Check sheet for the modelled part. Datum: model origin and axes. Units: mm. A direction names the side the tool comes from. Round coordinates to 2 decimals unless told otherwise and drop trailing zeros. Write each loop counter-clockwise with the first axis right and the second up, starting at its lowest first coordinate (ties: lowest second). Pieces come first, ordered by that corner, then holes. Notation, with made-up numbers: (76.5, -15) - (96.5, -15) arc R32 cw to (96.5, 15) - close; hole circle Ø5 at (39, 8.25). An arc over 180 degrees is marked (long way). Use one line per item in the form item = value. Start each with the question number.
1) Section check B-B (x = -83). Record the boundary of the cut face in (y, z).
2) Draft check along X on faces 1 (the face through (-90.14, -37.35, 19.32)), 2 (the face through (-110, -44.45, 16)), 3 (the face through (-31.433, -22, 6)). Enter one of: +X half, -X half, draft (parallel to the pull), parting line (faces both ways), or undercut.
3) Gauge pin test, flat ends, axial feed: P1, Ø8, axis at x = -94, y = -3, coming from the +Z side; P2, Ø5, axis at x = -149, y = -14, coming from the +Z side; P3, Ø1.5, axis at x = -154.5, y = -14, coming from the -Z side. Record the tip position at first contact, or that the pin passes through.
4) Section check A-A (y = -17.5). Record the boundary of the cut face in (x, z) (1 decimal), then the cut area to 3 significant figures.
5) Section check C-C (x = -56.5). Record the boundary of the cut face in (y, z), then the cut area to 3 significant figures.
6) Set-up check for faces 4 (the face through (-134.144, -22, 2)), 5 (the face through (-166.804, -29.652, 29.227)), 6 (the face through (-104, -41, 7.62)), 7 (the face through (-80, -7.62, 7)), 8 (the face through (-126.524, -23, 12)): record each of +Z, -Z, +X, -X, +Y, -Y from which the full face is reachable in a straight line by a thin tool's end or side.
7) Scan lines: probe 1 along Y at (x, z) = (-123, 2); probe 2 along X at (y, z) = (-12, 15). Record each from-to range of solid material in increasing order.
8) Section check D-D (z = 22). Record the boundary of the cut face in (x, y), then the cut area to 3 significant figures.
from build123d import *

# Parameters (mm, degrees)
F0_W      = 177.8
F0_H      = 44.45
F1_DEPTH  = 31.75
F2_W      = 1.5875
F2_H      = 44.45
F3_DEPTH  = 3.175
F4_W      = 95.09125
F4_H      = 29.21
F5_DEPTH  = 31.751
F7_DEPTH  = 44.451
F9_DEPTH  = 44.451
F11_DEPTH = 44.451
F13_DEPTH = 177.801
F14_R     = 2.54


with BuildPart() as f1:
    # F0 (on Top) → F1 (new body)
    with BuildSketch(Plane.XY):
        with Locations((-88.9, -22.225)):
            Rectangle(F0_W, F0_H)
    extrude(amount=F1_DEPTH)

    # F2 (on face) → F3 (cut)
    with BuildSketch(Plane(origin=(0, 0, 0), x_dir=(1, 0, 0), z_dir=(0, 0, -1))):
        with Locations((-23.01875, 22.225)):
            Rectangle(F2_W, F2_H)
        with Locations((-134.9375, 22.225)):
            Rectangle(F2_W, F2_H)
    extrude(amount=-F3_DEPTH, mode=Mode.SUBTRACT)

    # F4 (on face) → F5 (cut, through all)
    with BuildSketch(Plane.XY.offset(31.75)):
        with Locations((-78.978125, -22.225)):
            Rectangle(F4_W, F4_H)
    extrude(amount=-F5_DEPTH, mode=Mode.SUBTRACT)

    # F6 (on face) → F7 (cut, through all)
    with BuildSketch(Plane.XZ.offset(44.45)):
        Polygon((-177.8, 31.75), (0, 6.540501), (0, 31.75), align=None)
    extrude(amount=-F7_DEPTH, mode=Mode.SUBTRACT)

    # F8 (on face) → F9 (cut, through all)
    with BuildSketch(Plane.XZ.offset(44.45)):
        with BuildLine():
            Line((-126.52375, 16.783548), (-126.52375, 7.62))
            Line((-126.52375, 7.62), (-79.898132, 7.62))
            ThreePointArc((-79.898132, 7.62), (-78.63128, 8.800636), (-79.719847, 10.147424))
            Line((-79.719847, 10.147424), (-126.52375, 16.783548))
        make_face()
    extrude(amount=-F9_DEPTH, mode=Mode.SUBTRACT)

    # F10 (on face) → F11 (cut, through all)
    with BuildSketch(Plane.XZ.offset(44.45)):
        Polygon((-177.8, 0), (-148.43125, 0), (-177.8, 7.62), align=None)
    extrude(amount=-F11_DEPTH, mode=Mode.SUBTRACT)

    # F12 (on face) → F13 (cut, through all)
    with BuildSketch(Plane(origin=(-177.8, 0, 0), x_dir=(0, -1, 0), z_dir=(-1, 0, 0))):
        Polygon((41.121738, 31.75), (2.964308, 31.75), (22.565205, 27.667448), align=None)
    extrude(amount=-F13_DEPTH, mode=Mode.SUBTRACT)

    # F14
    f14_edges = [f1.edges().sort_by_distance(p)[0] for p in [
        (-31.4325, -36.83, 5.49859),
        (-126.52375, -36.83, 3.81),
        (-126.52375, -36.83, 20.631654),
        (-126.52375, -7.62, 3.81),
        (-126.52375, -7.62, 20.631654),
        (-31.4325, -7.62, 5.49859),
    ]]
    fillet(f14_edges, radius=F14_R)


solid = f1.part
Results are:
q1.outline = (-44.45, 0) - (-36.83, 0) - (-36.83, 7.62) - (-44.45, 7.62) - close; (-44.45, 10.61) - (-36.83, 10.61) - (-36.83, 18.31) - (-44.45, 18.31) - close; (-7.62, 0) - (0, 0) - (0, 7.62) - (-7.62, 7.62) - close; (-7.62, 10.61) - (0, 10.61) - (0, 18.31) - (-7.62, 18.31) - close
q2.face_1 = +X half
q2.face_2 = draft
q2.face_3 = undercut
q3.P1 = 20.44
q3.P2 = 28.02
q3.P3 = 1.38
q4.outline = (-177.8, 7.6) - (-148.4, 0) - (-135.7, 0) - (-135.7, 3.2) - (-134.1, 3.2) - (-134.1, 0) - (-126.5, 0) - (-126.5, 24.5) - (-156.4, 28.7) - (-177.8, 28.7) - close; (-31.4, 0) - (-23.8, 0) - (-23.8, 3.2) - (-22.2, 3.2) - (-22.2, 0) - (0, 0) - (0, 6.5) - (-31.4, 11) - close
q4.area = 1,560 mm²
q5.outline = (-44.45, 0) - (-36.83, 0) - (-36.83, 14.55) - (-44.45, 14.55) - close; (-7.62, 0) - (0, 0) - (0, 14.55) - (-7.62, 14.55) - close
q5.area = 222 mm²
q6.face_4 = -Z, +Y, -Y
q6.face_5 = +Z, +X, -X
q6.face_6 = +Y, -Y
q6.face_7 = +Z, -Z
q6.face_8 = none
q7.probe_1 = -44.45 to -36.83, -7.62 to 0
q7.probe_2 = -177.8 to -126.52
q8.outline = (-177.8, -44.45) - (-109.03, -44.45) - (-109.03, -36.83) - (-123.98, -36.83) arc R2.54 cw to (-126.52, -34.29) - (-126.52, -10.16) arc R2.54 cw to (-123.98, -7.62) - (-109.03, -7.62) - (-109.03, 0) - (-177.8, 0) - close
q8.area = 2,550 mm²
